Can you work these out from the drawing? Everything is in mm from the part's minimum corner. A direction names the side the tool comes from. Give positions to 0.01 mm unless a question says otherwise; leave off trailing zeros. Write each loop counter-clockwise with the first axis right and the second up, starting at its lowest first coordinate (ties: lowest second). Pieces come first, ordered by that corner, then holes. Notation, with made-up numbers: (56, 37.5) - (85, 37.5) arc R12 ccw to (85, 48.5) - close; hole circle Ø5 at (2.5, 64). An arc over 180 degrees is marked (long way). Answer in a Markdown table with one row per item.
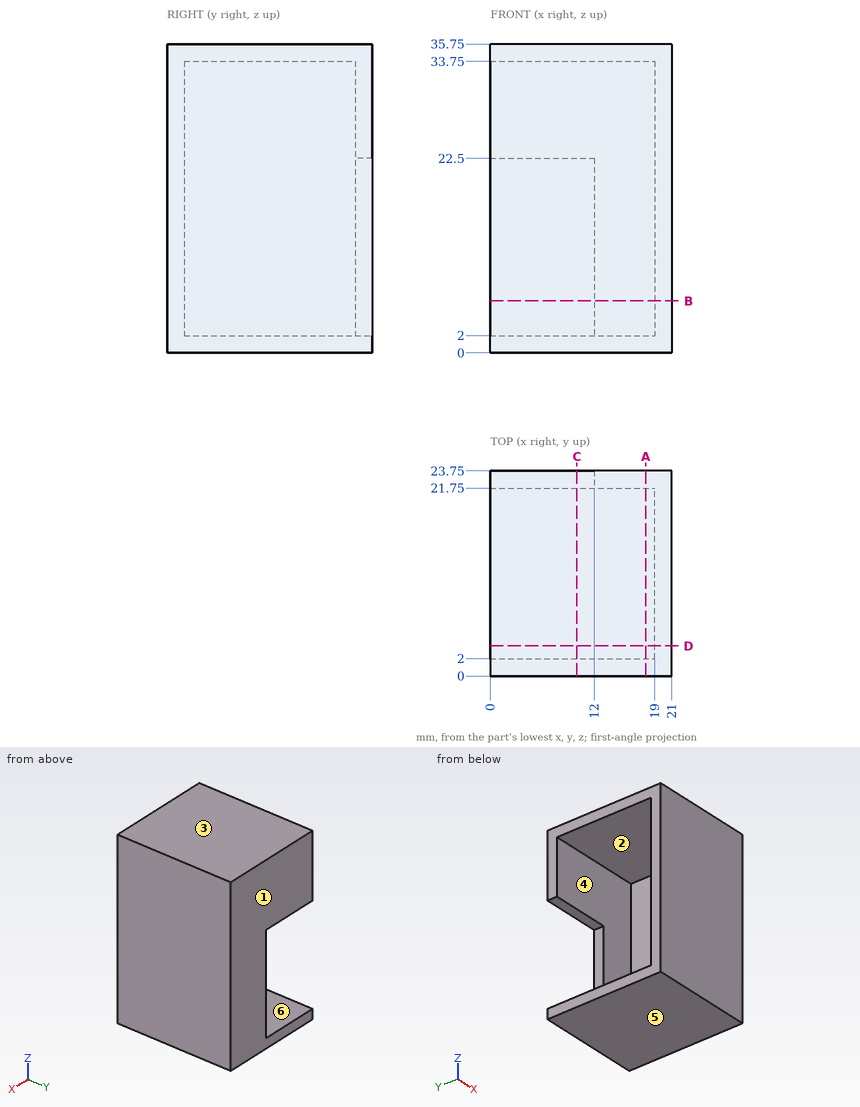
1) Imagine slicing it at B-B (z = 6). List the corners of the cut face in (x, y) for me.
Check values:
| item | result |
|---|---|
| outline | (0, 0) - (21, 0) - (21, 23.75) - (12, 23.75) - (12, 21.75) - (19, 21.75) - (19, 2) - (0, 2) - close |
2) We'd pull the mould along Z, two halves only. Please class the marked faces 1, 2, 3 and 4: +Z half, -Z half, draft (parallel to the pull), parting line (faces both ways), or undercut.
Check values:
| item | result |
|---|---|
| face 1 | draft |
| face 2 | undercut |
| face 3 | +Z half |
| face 4 | undercut |
3) Imagine slicing it at C-C (x = 10). List the corners of the cut face in (y, z) for me.
Check values:
| item | result |
|---|---|
| outline | (0, 0) - (23.75, 0) - (23.75, 2) - (2, 2) - (2, 33.75) - (21.75, 33.75) - (21.75, 22.5) - (23.75, 22.5) - (23.75, 35.75) - (0, 35.75) - close |
4) Imagine slicing it at A-A (x = 18). List the corners of the cut face in (y, z) for me.
Check values:
| item | result |
|---|---|
| outline | (0, 0) - (23.75, 0) - (23.75, 35.75) - (0, 35.75) - close; hole (2, 2) - (21.75, 2) - (21.75, 33.75) - (2, 33.75) - close |
5) Will these pins go through, and if not, where does the flat tip stop? P1, Ø3, axis at x = 7.5, z = 14, coming from the +Y side; P2, Ø1, axis at y = 22.5, z = 10, coming from the -X side; P3, Ø10, axis at y = 10.5, z = 15.5, coming from the -X side.
Check values:
| item | result |
|---|---|
| P1 | stops at y = 2 |
| P2 | stops at x = 12 |
| P3 | stops at x = 19 |
6) If I drill on line 1 (Z direction, x = 14.75, y = 19); line 2 (Y direction, x = 7.75, z = 33); line 3 (X direction, y = 9.5, z = 26.5), over which ranges is the centre line in solid material (lowest first)?
Check values:
| item | result |
|---|---|
| line 1 | z = 0 to 2, 33.75 to 35.75 |
| line 2 | y = 0 to 2, 21.75 to 23.75 |
| line 3 | x = 19 to 21 |
7) Imagine slicing it at D-D (y = 3.5). List the corners of the cut face in (x, z) for me, then the cut area to 4 significant figures.
Check values:
| item | result |
|---|---|
| outline | (0, 0) - (21, 0) - (21, 35.75) - (0, 35.75) - (0, 33.75) - (19, 33.75) - (19, 2) - (0, 2) - close |
| area | 147.5 mm2 |
8) On a 3-axis mill with a long thin cutter (end or side, diameter ignored), from which of +Z, -Z, +X, -X, +Y, -Y can I reach the whole of each face in a straight line? I mean the marked faces 5 and 6. Say none if no direction works.
Check values:
| item | result |
|---|---|
| face 5 | -Z, +X, -X, +Y, -Y |
| face 6 | -X |
